```python
from build123d import *

# Parameters (mm, degrees)
F1_DEPTH = 16
F5_R     = 2.5
F6_DEPTH = 10
F7_R     = 5
F8_DEPTH = 10


with BuildPart() as f1:
    # F0 (on Top) → F1 (new body)
    with BuildSketch(Plane.XY):
        with BuildLine():
            Line((-7.5, 4.974937), (-7.5, -4.974937))
            ThreePointArc((-7.5, -4.974937), (0, -9), (7.5, -4.974937))
            Line((7.5, -4.974937), (7.5, 4.974937))
            ThreePointArc((7.5, 4.974937), (0, 9), (-7.5, 4.974937))
        make_face()
    extrude(amount=F1_DEPTH)



with BuildPart() as f4:
    # F3 (on offset) → F4 (revolve)
    with BuildSketch(Plane.XY.offset(26)):
        with BuildLine():
            Line((0, -5), (0, 5))
            ThreePointArc((0, 5), (-5, 0), (0, -5))
        make_face()
    revolve(axis=Axis((0, 0, 26), (0, -1, 0)))


with BuildPart() as f1_1:
    add(f1.part)

    add(f4.part)  # F6 merges F4
    # F5 (on face) → F6 (join)
    with BuildSketch(Plane.XY.offset(16)):
        Circle(F5_R)
    extrude(amount=F6_DEPTH)

    # F7 (on face) → F8 (cut)
    with BuildSketch(Plane(origin=(0, 0, 0), x_dir=(1, 0, 0), z_dir=(0, 0, -1))):
        Circle(F7_R)
    extrude(amount=-F8_DEPTH, mode=Mode.SUBTRACT)


solid = f1_1.part
```
Verification items for the finished model (mm, model axes). A direction names the side the tool comes from. Round coordinates to 2 decimals unless told otherwise and drop trailing zeros. Order: outer loops, then holes, each group sorted by start corner. A loop starts at its lowest first (then second) coordinate and runs counter-clockwise, first axis right, second up. Notation, with made-up numbers: (27.5, -19.5) -> (59.5, -19.5) arc R23 cw to (59.5, 11.5) -> close; hole circle Ø4 at (-24, -8.5). An arc over 180 degrees is marked (long way). Put each result on its own line as item: value. Start each with the question number.
(1) Depth check by flat-ended pin: pin 1 Ø1 at (x, y) = (-2.5, -6) entering from +Z; pin 2 Ø1.5 at (y, z) = (2, 27.5) entering from +X; pin 3 Ø1.5 at (y, z) = (-4.5, 27) entering from +X. Enter the tip coordinate at first touch or a pass-through.
(2) Section check D-D (y = 0). Enter the section's corners in (x, z), then the cut area to 3 significant figures.
(3) Section check C-C (x = 0). Enter the section's corners in (y, z), then the cut area to 3 significant figures.
(4) Draft check along Y on faces 1 (the face through (-7.5, 0, 8)), 2 (the face through (0, 9, 8)), 3 (the face through (0, 0, 10)). Enter one of: +Y half, -Y half, draft (parallel to the pull), parting line (faces both ways), or undercut.
(5) Section check B-B (z = 8). Enter the section's corners in (x, y), then the cut area to 3 significant figures.
(6) Section check A-A (y = 3.5). Enter the section's corners in (x, z).
(7) Tool access check on faces 4 (the face through (-1.08, 4.88, 4.93)), 5 (the face through (7.5, 0, 8)), 6 (the face through (2, 2, 16)). Record the directions out of +Z, -Z, +X, -X, +Y, -Y that give a thin tool (end or side, any length) a straight path to the whole face; none if there is none.
(8) Material ranges on line 1 along X through (y, z) = (0, 7.5); line 2 along Z through (x, y) = (-5.5, -2.25); line 3 along Y through (x, z) = (-4.5, 2), recorded low to high.
Completed:
1. pin 1: stops at z = 16
1. pin 2: stops at x = 4.68
1. pin 3: stops at x = 3.18
2. outline: (-7.5, 0) -> (-5, 0) -> (-5, 10) -> (5, 10) -> (5, 0) -> (7.5, 0) -> (7.5, 16) -> (2.5, 16) -> (2.5, 21.67) arc R5 ccw (long way) to (-2.5, 21.67) -> (-2.5, 16) -> (-7.5, 16) -> close
2. area: 245 mm2
3. outline: (-9, 0) -> (-5, 0) -> (-5, 10) -> (5, 10) -> (5, 0) -> (9, 0) -> (9, 16) -> (2.5, 16) -> (2.5, 21.67) arc R5 ccw (long way) to (-2.5, 21.67) -> (-2.5, 16) -> (-9, 16) -> close
3. area: 293 mm2
4. face 1: draft
4. face 2: +Y half
4. face 3: undercut
5. outline: (-7.5, -4.97) arc R9 ccw to (7.5, -4.97) -> (7.5, 4.97) arc R9 ccw to (-7.5, 4.97) -> close; hole circle Ø10 at (0, 0)
5. area: 156 mm2
6. outline: (-7.5, 0) -> (-3.57, 0) -> (-3.57, 10) -> (3.57, 10) -> (3.57, 0) -> (7.5, 0) -> (7.5, 16) -> (-7.5, 16) -> close; circle Ø7.14 at (0, 26)
7. face 4: -Z
7. face 5: +Z, -Z, +X, +Y, -Y
7. face 6: none
8. line 1: x = -7.5 to -5, 5 to 7.5
8. line 2: z = 0 to 16
8. line 3: y = -7.79 to -2.18, 2.18 to 7.79
